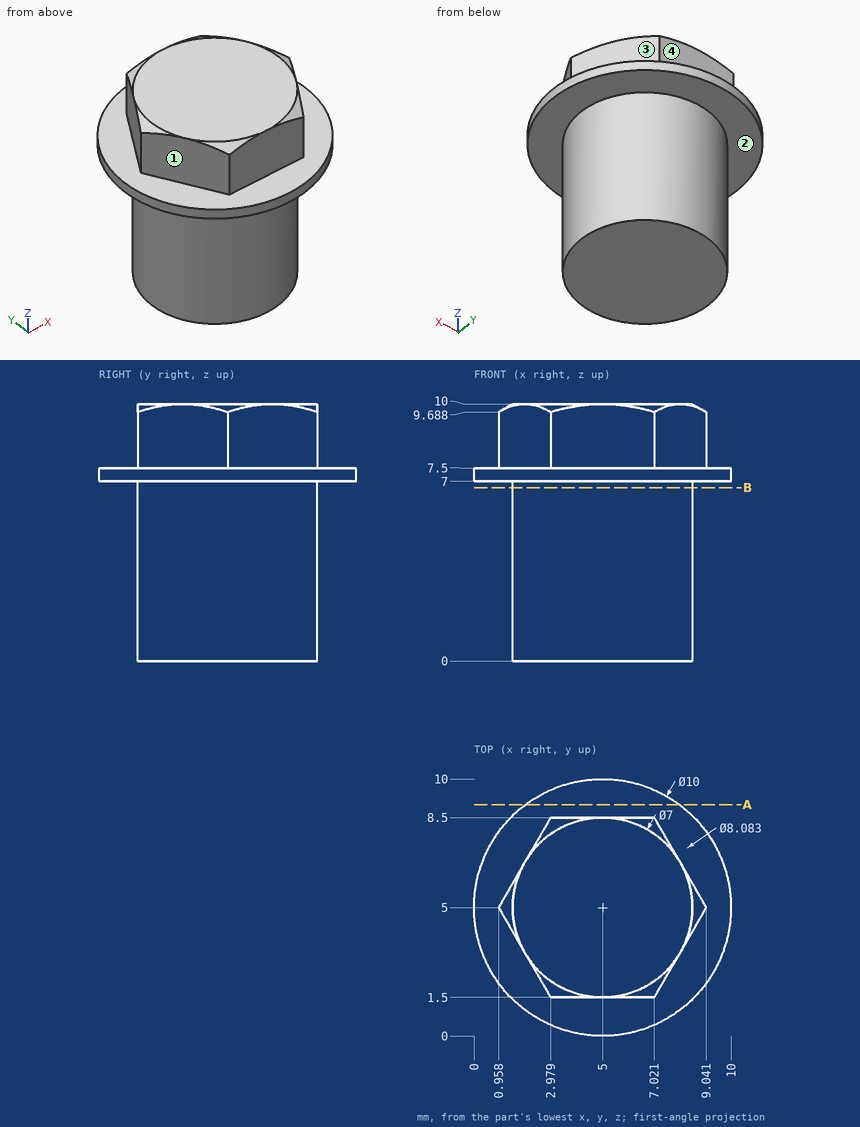
Could you check a few things on this drawing? It's one solid part, dimensions in mm from its lowest x, y, z. A direction names the side the tool comes from. Give positions to 0.01 mm unless a question says otherwise; leave off trailing zeros. Order: outer loops, then holes, each group sorted by start corner. A loop starts at its lowest first (then second) coordinate and runs counter-clockwise, first axis right, second up. Notation, with made-up numbers: (9.25, -24.5) -> (17.25, -24.5) arc R27 cw to (17.25, 0.5) -> close; hole circle Ø3 at (33, 74). An arc over 180 degrees is marked (long way). Answer in a Markdown table with one row per item. Add a question column.
Item 1: I'm going to push flat-ended pins straight in: P1, Ø1.5, axis at x = 5, z = 5, coming from the -Y side; P2, Ø6, axis at y = 4, z = 1.5, coming from the +X side; P3, Ø1.2, axis at x = 4, z = 9, coming from the +Y side. Where does each tip first touch, or does it pass through?
Item 2: For the marked faces 1, 2, 3 and 4, which set-ups out of +Z, -Z, +X, -X, +Y, -Y let a thin tool reach every point of the face, with its end or its side?
Item 3: Imagine slicing it at A-A (y = 9). List the corners of the cut face in (x, z) for me.
Item 4: Please list where these lines run through material, in increasing order: probe 1 along Z at (x, y) = (8.75, 2.75); probe 2 along Y at (x, z) = (5, 8); probe 3 along X at (y, z) = (7.5, 4.5).
Item 5: Imagine slicing it at B-B (z = 6.75). List the corners of the cut face in (x, y) for me, and give its area (3 significant figures).
Result:
| question | item | result |
|---|---|---|
| 1 | P1 | y = 1.5 |
| 1 | P2 | x = 8.5 |
| 1 | P3 | y = 8.5 |
| 2 | face 1 | +Z, -X, -Y |
| 2 | face 2 | -Z |
| 2 | face 3 | +Z, +X, +Y |
| 2 | face 4 | +Z, +X, -X, +Y |
| 3 | outline | (2, 7) -> (8, 7) -> (8, 7.5) -> (2, 7.5) -> close |
| 4 | probe 1 | 7 to 7.5 |
| 4 | probe 2 | 1.5 to 8.5 |
| 4 | probe 3 | 2.55 to 7.45 |
| 5 | outline | circle Ø7 at (5, 5) |
| 5 | area | 38.5 mm2 |
